Design review of the part built by this model. Coordinates are the model's own, in mm. A direction names the side the tool comes from. Give positions to 0.01 mm unless a question says otherwise; leave off trailing zeros. Order: outer loops, then holes, each group sorted by start corner. A loop starts at its lowest first (then second) coordinate and runs counter-clockwise, first axis right, second up. Notation, with made-up numbers: (82, -33.5) -> (129, -33.5) arc R17 cw to (129, -23.5) -> close; hole circle Ø7 at (64, 33). An arc over 180 degrees is marked (long way). Answer in a Markdown table with one row per item. Add a question column.
```python
from build123d import *

# Parameters (mm, degrees)
BOSS_EXTRUDE1_DEPTH                             = 36.5
CUT_EXTRUDE1_DEPTH                              = 32.5
CUT_EXTRUDE1_DEPTH_BACK                         = 32.5
SKETCH2_W                                       = 30
SKETCH2_H                                       = 65
CUT_EXTRUDE2_DEPTH                              = 84.447588341
CUT_EXTRUDE2_DEPTH_BACK                         = 84.447588341
SKETCH3_R                                       = 11.25
SKETCH4_R                                       = 11.25
SKETCH4_R_2                                     = 9.75
BOSS_EXTRUDE2_DEPTH                             = 2
TAP_DRILL_FOR_M3X0_5_TAP1_D                     = 2.5
CSK_FOR_M3_FLAT_HEAD_MACHINE_SCREW1_D           = 3.2
CSK_FOR_M3_FLAT_HEAD_MACHINE_SCREW1_DEPTH       = 8
CSK_FOR_M3_FLAT_HEAD_MACHINE_SCREW1_CSINK_D     = 6.3
CSK_FOR_M3_FLAT_HEAD_MACHINE_SCREW1_CSINK_ANGLE = 90
CUT_EXTRUDE4_DEPTH                              = 84.447588341
CUT_EXTRUDE4_DEPTH_BACK                         = 84.447588341
CHAMFER1_SIZE                                   = 0.5
BOSS_EXTRUDE3_START                             = -34
SKETCH4_2_R                                     = 11.25
SKETCH4_2_R_2                                   = 9.75
BOSS_EXTRUDE3_DEPTH                             = 4
M3_CLEARANCE_HOLE1_D                            = 3.6
M3_CLEARANCE_HOLE1_DEPTH                        = 8
CUT_EXTRUDE3_DEPTH                              = 99.905257696
CHAMFER2_SIZE                                   = 1
CHAMFER2_OF_MIRROR1_SIZE                        = 1


with BuildPart() as part:
    # Sketch1 → Boss-Extrude1 (new, symmetric)
    with BuildSketch(Plane.XY):
        Polygon((-8, 32.5), (-8, -22.5), (-18, -32.5), (-28, -32.5), (-38, -22.5), (-38, 32.5), (-46, 32.5), (-46, -37.5), (65, -37.5), (65, -32.5), (0, 32.5), align=None)
    extrude(amount=BOSS_EXTRUDE1_DEPTH, both=True)

    # Sketch2 → Cut-Extrude1 (cut, two sides: drawn at the far end of the back side and taken through both)
    with BuildSketch(Plane.XY.offset(-CUT_EXTRUDE1_DEPTH_BACK)):
        with Locations((-23, 0)):
            Rectangle(SKETCH2_W, SKETCH2_H)
        Polygon((0, 32.5), (0, -32.5), (65, -32.5), align=None)
    extrude(amount=CUT_EXTRUDE1_DEPTH + CUT_EXTRUDE1_DEPTH_BACK, mode=Mode.SUBTRACT)

    # Sketch3 → Cut-Extrude2 (cut, two sides: drawn at the far end of the back side and taken through both)
    with BuildSketch(Plane(origin=(0, 0, 0), x_dir=(0, 0, -1), z_dir=(1, 0, 0)).offset(-CUT_EXTRUDE2_DEPTH_BACK)):
        with Locations(Location((0, 0, 0), (0, 0, 90))):
            Circle(SKETCH3_R)
    extrude(amount=CUT_EXTRUDE2_DEPTH + CUT_EXTRUDE2_DEPTH_BACK, mode=Mode.SUBTRACT)

    # Sketch4 → Boss-Extrude2 (add)
    with BuildSketch(Plane.ZY.offset(38)):
        with Locations(Location((0, 0, 0), (0, 0, 90))):
            Circle(SKETCH4_R)
        with Locations(Location((0, 0, 0), (0, 0, 270))):
            Circle(SKETCH4_R_2, mode=Mode.SUBTRACT)
    extrude(amount=BOSS_EXTRUDE2_DEPTH)

    # Tap Drill for M3x0.5 Tap1 (through all)
    with Locations(Plane.ZY.offset(46)):
        with Locations((-9.545941546, 9.545941546), (9.545941546, -9.545941546)):
            Hole(TAP_DRILL_FOR_M3X0_5_TAP1_D / 2)

    # CSK for M3 Flat Head Machine Screw1
    with Locations(Plane.ZY.offset(8)):
        with Locations((-23.5, 23.5), (23.5, 23.5), (23.5, -23.5), (-23.5, -23.5), (0, 0)):
            CounterSinkHole(CSK_FOR_M3_FLAT_HEAD_MACHINE_SCREW1_D / 2, CSK_FOR_M3_FLAT_HEAD_MACHINE_SCREW1_CSINK_D / 2, depth=CSK_FOR_M3_FLAT_HEAD_MACHINE_SCREW1_DEPTH, counter_sink_angle=CSK_FOR_M3_FLAT_HEAD_MACHINE_SCREW1_CSINK_ANGLE)

    # Sketch21 → Cut-Extrude4 (cut, two sides: drawn at the far end of the back side and taken through both)
    with BuildSketch(Plane.XY.offset(-CUT_EXTRUDE4_DEPTH_BACK)):
        Polygon((-5, -37.5), (-4, -35.5), (-3, -37.5), align=None)
    extrude(amount=CUT_EXTRUDE4_DEPTH + CUT_EXTRUDE4_DEPTH_BACK, mode=Mode.SUBTRACT)

    # Chamfer1
    chamfer1_edges = [part.edges().sort_by_distance(p)[0] for p in [
        (0, -11.25, 0),
        (-46, -11.25, 0),
        (-8, -27.5, -32.5),
        (-8, -27.5, 32.5),
        (-13, -32.5, 32.5),
        (-8, -32.5, 0),
        (-13, -32.5, -32.5),
        (-38, -27.5, 32.5),
        (-38, -27.5, -32.5),
        (-33, -32.5, -32.5),
        (-38, -32.5, 0),
        (-33, -32.5, 32.5),
        (32.5, -32.5, 32.5),
        (0, -32.5, 0),
        (32.5, -32.5, -32.5),
        (0, 32.5, 0),
        (-8, 32.5, 0),
        (-4, 32.5, 36.5),
        (-8, 5, 36.5),
        (-13, -27.5, 36.5),
        (-23, -32.5, 36.5),
        (-33, -27.5, 36.5),
        (-38, 5, 36.5),
        (-42, 32.5, 36.5),
        (-38, 32.5, 0),
        (-46, 32.5, 0),
        (-42, 32.5, -36.5),
        (-38, 5, -36.5),
        (-33, -27.5, -36.5),
        (-23, -32.5, -36.5),
        (-13, -27.5, -36.5),
        (-8, 5, -36.5),
        (-4, 32.5, -36.5),
        (32.5, 0, 36.5),
        (32.5, 0, -36.5),
        (65, -35, 36.5),
        (65, -35, -36.5),
        (-46, -2.5, -36.5),
        (-46, -2.5, 36.5),
        (65, -37.5, 0),
        (-25.5, -37.5, -36.5),
        (31, -37.5, -36.5),
        (-46, -37.5, 0),
        (31, -37.5, 36.5),
        (-25.5, -37.5, 36.5),
    ]]
    chamfer(chamfer1_edges, length=CHAMFER1_SIZE)

    # Sketch4<2> → Boss-Extrude3 (add)
    with BuildSketch(Plane.ZY.offset(38).offset(BOSS_EXTRUDE3_START)):
        with Locations(Location((0, 0, 0), (0, 0, 180))):
            Circle(SKETCH4_2_R)
        with Locations(Location((0, 0, 0), (0, 0, 270))):
            Circle(SKETCH4_2_R_2, mode=Mode.SUBTRACT)
    extrude(amount=BOSS_EXTRUDE3_DEPTH)

    # M3 Clearance Hole1
    with Locations(Plane.ZY.offset(46)):
        with Locations((-23.5, -23.5), (23.5, -23.5), (23.5, 23.5), (-23.5, 23.5)):
            Hole(M3_CLEARANCE_HOLE1_D / 2, depth=M3_CLEARANCE_HOLE1_DEPTH)

    # Sketch19 → Cut-Extrude3 (cut, through all)
    with BuildSketch(Plane(origin=(0, -32.5, 0), x_dir=(1, 0, 0), z_dir=(0, 1, 0))):
        with BuildLine():
            Line((-34, 5), (-34, 27.5))
            ThreePointArc((-34, 27.5), (-32, 29.5), (-30, 27.5))
            Line((-30, 27.5), (-30, 5))
            ThreePointArc((-30, 5), (-32, 3), (-34, 5))
        make_face()
        with BuildLine():
            Line((-16, 5), (-16, 27.5))
            ThreePointArc((-16, 27.5), (-14, 29.5), (-12, 27.5))
            Line((-12, 27.5), (-12, 5))
            ThreePointArc((-12, 5), (-14, 3), (-16, 5))
        make_face()
        with BuildLine():
            Line((6, 5), (6, 27.5))
            ThreePointArc((6, 27.5), (8, 29.5), (10, 27.5))
            Line((10, 27.5), (10, 5))
            ThreePointArc((10, 5), (8, 3), (6, 5))
        make_face()
        with BuildLine():
            Line((55, 5), (55, 27.5))
            ThreePointArc((55, 27.5), (57, 29.5), (59, 27.5))
            Line((59, 27.5), (59, 5))
            ThreePointArc((59, 5), (57, 3), (55, 5))
        make_face()
    cut_extrude3 = extrude(amount=-CUT_EXTRUDE3_DEPTH, mode=Mode.SUBTRACT)

    # Chamfer2
    chamfer2_edges = [part.edges().sort_by_distance(p)[0] for p in [
        (-32, -32.5, -3),
        (-30, -32.5, -16.25),
        (-32, -32.5, -29.5),
        (-34, -32.5, -16.25),
        (-14, -32.5, -3),
        (-12, -32.5, -16.25),
        (-14, -32.5, -29.5),
        (-16, -32.5, -16.25),
        (8, -32.5, -3),
        (10, -32.5, -16.25),
        (8, -32.5, -29.5),
        (6, -32.5, -16.25),
        (57, -32.5, -3),
        (59, -32.5, -16.25),
        (57, -32.5, -29.5),
        (55, -32.5, -16.25),
    ]]
    chamfer(chamfer2_edges, length=CHAMFER2_SIZE)

    # Mirror1: Cut-Extrude3 across plane
    add(cut_extrude3.mirror(Plane.XY), mode=Mode.SUBTRACT)

    # Chamfer2 of Mirror1
    chamfer2_of_mirror1_edges = [part.edges().sort_by_distance(p)[0] for p in [
        (-32, -32.5, 3),
        (-30, -32.5, 16.25),
        (-32, -32.5, 29.5),
        (-34, -32.5, 16.25),
        (-14, -32.5, 3),
        (-12, -32.5, 16.25),
        (-14, -32.5, 29.5),
        (-16, -32.5, 16.25),
        (8, -32.5, 3),
        (10, -32.5, 16.25),
        (8, -32.5, 29.5),
        (6, -32.5, 16.25),
        (57, -32.5, 3),
        (59, -32.5, 16.25),
        (57, -32.5, 29.5),
        (55, -32.5, 16.25),
    ]]
    chamfer(chamfer2_of_mirror1_edges, length=CHAMFER2_OF_MIRROR1_SIZE)


solid = part.part
```
1) Clearance check with flat-ended pins moving along their axes: P1, Ø11.5, axis at y = 0, z = 0, coming from the -X side; P2, Ø19, axis at y = 14.5, z = -12, coming from the +X side; P3, Ø6, axis at x = 36.5, z = 26, coming from the +Y side. State where each tip first meets the part, or that it passes through.
2) Add section A-A, the plane x = 8. Write out the cut boundary in (y, z), and give its area (3 significant figures).
3) Mouldability with a two-part tool opening along X and no side actions: class faces 1 (the face through (32, -32.5, 0)), 2 (the face through (55, -35, -16)) as +X half, -X half, draft (parallel to the pull), parting line (faces both ways), or undercut.
4) Machinability: for faces 3 (the face through (-12, -35, -16)), 4 (the face through (-32, -33.3, -2.8)), 5 (the face through (-12.9, -27.4, -34.4)), which of the approach directions +Z, -Z, +X, -X, +Y, -Y give a long, thin tool a straight path to every point of the face, cutting with its end or side? Answer none if there is none.
5) Add section D-D, the plane x = 36. Write out the cut boundary in (y, z).
6) Add section C-C, the plane y = -19. Write out the cut boundary in (x, z).
7) For L1, parallel to X at y = -34.5, z = 20; L2, parallel to Y at x = -40.25, z = 23.5; L3, parallel to Z at x = 31, y = -13, list the stretches that pass through material, from the lowest coordinate up.
8) Add section B-B, the plane z = 0. Give the number of separate pieces and of enclosed holes in the cut face, and give its area (3 significant figures).
Verdict:
| question | item | result |
|---|---|---|
| 1 | P1 | passes through |
| 1 | P2 | stops at x = 0 |
| 1 | P3 | stops at y = -32.5 |
| 2 | outline | (-37.5, -36) -> (-37, -36.5) -> (23.79, -36.5) -> (24.5, -36) -> (24.5, -32.5) -> (-32, -32.5) -> (-32.5, -32) -> (-32.5, -30.5) -> (-33.5, -29.5) -> (-37.5, -29.5) -> close; (-37.5, -3) -> (-33.5, -3) -> (-32.5, -2) -> (-32.5, 2) -> (-33.5, 3) -> (-37.5, 3) -> close; (-37.5, 29.5) -> (-33.5, 29.5) -> (-32.5, 30.5) -> (-32.5, 32) -> (-32, 32.5) -> (24.5, 32.5) -> (24.5, 36) -> (23.79, 36.5) -> (-37, 36.5) -> (-37.5, 36) -> close |
| 2 | area | 554 mm2 |
| 3 | face 1 | draft |
| 3 | face 2 | undercut |
| 4 | face 3 | +Y, -Y |
| 4 | face 4 | +Y |
| 4 | face 5 | +Z, -Z, +Y |
| 5 | outline | (-37.5, -36) -> (-37, -36.5) -> (-4.21, -36.5) -> (-3.5, -36) -> (-3.5, -32.5) -> (-32, -32.5) -> (-32.5, -32) -> (-32.5, 32) -> (-32, 32.5) -> (-3.5, 32.5) -> (-3.5, 36) -> (-4.21, 36.5) -> (-37, 36.5) -> (-37.5, 36) -> close |
| 6 | outline | (-46, -36) -> (-45.5, -36.5) -> (-38.5, -36.5) -> (-38, -36) -> (-38, 36) -> (-38.5, 36.5) -> (-45.5, 36.5) -> (-46, 36) -> close; (-8, -36) -> (-7.5, -36.5) -> (50.79, -36.5) -> (51.5, -36) -> (51.5, -32.5) -> (0, -32.5) -> (0, 32.5) -> (51.5, 32.5) -> (51.5, 36) -> (50.79, 36.5) -> (-7.5, 36.5) -> (-8, 36) -> close |
| 7 | L1 | x = -46 to -34, -30 to -16, -12 to 6, 10 to 55, 59 to 65 |
| 7 | L2 | y = -37.5 to -25.3, -21.7 to 21.7, 25.3 to 32.5 |
| 7 | L3 | z = -36.5 to -32.5, 32.5 to 36.5 |
| 8 | separate pieces | 3 |
| 8 | enclosed holes | 0 |
| 8 | area | 1,250 mm2 |
